Work out the finished part from the listing and answer in its coordinate system (mm). Face numbers are marked on the shaded views. A direction names the side the tool comes from. Give positions to 0.01 mm unless a question says otherwise; leave off trailing zeros. Order: outer loops, then holes, each group sorted by start corner. A loop starts at its lowest first (then second) coordinate and runs counter-clockwise, first axis right, second up. Notation, with made-up numbers: (40.25, 35.5) -> (97.25, 35.5) arc R16 ccw to (97.25, 55.5) -> close; hole circle Ø3 at (87, 11.25). An arc over 180 degrees is marked (long way). Answer as CSV lines item,"result". Start each with the question number.
1. A cutting plane is placed at B-B (y = 11.5). Give the vertices of the cut face in (x, z).
2. For the marked faces 4 and 5, determine the directions among +Z, -Z, +X, -X, +Y, -Y from which every point of the face is accessible in a straight line to the end or side of a thin tool.
3. Find the intervals of material crossed by L1, parallel to Y at x = 138, z = -21; L2, parallel to X at y = 10.5, z = -10; L3, parallel to Y at x = 9, z = -15.5, in increasing order.
4. A cutting plane is placed at A-A (x = 27). Give the vertices of the cut face in (y, z), then the cut area to 3 significant figures.
5. For a pull along X with two mould halves and no side action, classify the marked faces 1, 2 and 3 as released by +X, released by -X, zero draft, split by the parting line, or undercut.
6. Flat-ended cylindrical pins translate along their axes: pin 1 (10 mm diameter, centred on x = 104, z = -6, fed in from -Y); pin 2 (6 mm diameter, centred on x = 30.5, z = -6.5, fed in from +Y); pin 3 (4.5 mm diameter, centred on y = 10.5, z = -31.5, fed in from +X). Find the tip coordinate at first contact, or state that the pin passes through.
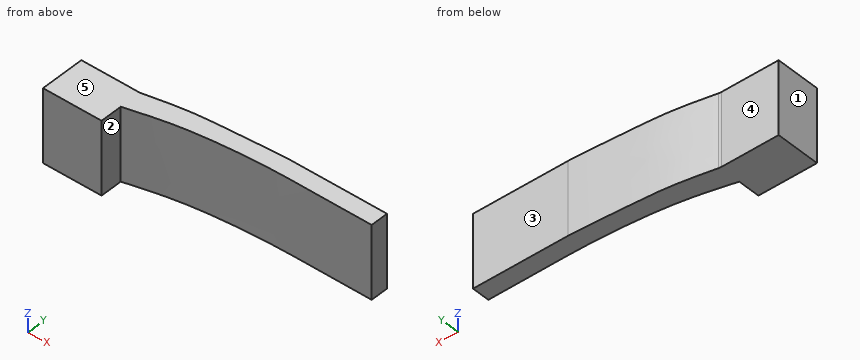
from build123d import *

# Parameters (mm, degrees)
SKETCH1_W           = 200
SKETCH1_H           = 50
BOSS_EXTRUDE1_DEPTH = 40
CUT_EXTRUDE1_DEPTH  = 51
CUT_EXTRUDE2_DEPTH  = 51.0000001
FILLET3_R           = 10


with BuildPart() as part:
    # Sketch1 → Boss-Extrude1 (new body)
    with BuildSketch(Plane(origin=(0, 0, 0), x_dir=(1, 0, 0), z_dir=(0, 1, 0))):
        with Locations((100, 25)):
            Rectangle(SKETCH1_W, SKETCH1_H)
    extrude(amount=BOSS_EXTRUDE1_DEPTH)

    # Sketch9 → Cut-Extrude1 (cut, through all)
    with BuildSketch(Plane.XY):
        with BuildLine():
            Line((40, 15), (40, 0))
            Line((40, 0), (200, 0))
            Line((200, 0), (200, 28))
            add(Edge.make_bspline(
                [(40, 15), (49.956623556, 17.554557146), (69.695225932, 22.618863079), (101.569485276, 26.484663085), (134.972625039, 28.43029981), (168.335074049, 27.910219147), (190.0005497, 27.971648152), (200, 28)],
                knots=[0, 0, 0, 0, 0.19118813, 0.379022714, 0.596595093, 0.81381312, 1, 1, 1, 1], degree=3))
        make_face()
    extrude(amount=-CUT_EXTRUDE1_DEPTH, mode=Mode.SUBTRACT)

    # Sketch11 → Cut-Extrude2 (cut, through all)
    with BuildSketch(Plane.XY):
        with BuildLine():
            Line((0, 30), (40, 30))
            add(Edge.make_bspline(
                [(40, 30), (49.965685719, 32.090607049), (69.767662187, 36.244676598), (101.665880925, 37.991623988), (123.327031089, 39.644618931), (135, 40)],
                knots=[0, 0, 0, 0, 0.233428343, 0.46382584, 0.73213141, 0.73213141, 0.73213141, 0.73213141], degree=3))
            Line((135, 40), (0, 40))
            Line((0, 40), (0, 30))
        make_face()
    extrude(amount=-CUT_EXTRUDE2_DEPTH, mode=Mode.SUBTRACT)

    # Fillet3
    fillet3_edges = [part.edges().sort_by_distance(p)[0] for p in [
        (40, 30, -25),
    ]]
    fillet(fillet3_edges, radius=FILLET3_R)


solid = part.part
Answer sheet:
1,outline,"(0, -50) -> (40, -50) -> (40, 0) -> (0, 0) -> close"
2,face 4,"+Z, -Z, -X, +Y"
2,face 5,"+Z, +X, -X, +Y, -Y"
3,L1,"y = 28.05 to 40"
3,L2,"x = 0 to 40"
3,L3,"y = 0 to 30"
4,outline,"(0, -50) -> (30, -50) -> (30, 0) -> (0, 0) -> close"
4,area,"1,500 mm^2"
5,face 1,"released by -X"
5,face 2,"released by +X"
5,face 3,"zero draft"
6,pin 1,"stops at y = 25.91"
6,pin 2,"stops at y = 30"
6,pin 3,"stops at x = 40"
